from build123d import *

# Parameters (mm, degrees)
SKETCH1_W           = 87
SKETCH1_H           = 90
BOSS_EXTRUDE1_DEPTH = 3
SKETCH2_R           = 3
CUT_EXTRUDE1_DEPTH  = 63.659795723
SKETCH3_R           = 3
CUT_EXTRUDE2_DEPTH  = 63.659795723


with BuildPart() as part:
    # Sketch1 → Boss-Extrude1 (new body)
    with BuildSketch(Plane(origin=(0, 0, 0), x_dir=(1, 0, 0), z_dir=(0, 1, 0))):
        Rectangle(SKETCH1_W, SKETCH1_H)
    extrude(amount=BOSS_EXTRUDE1_DEPTH)

    # Sketch2 → Cut-Extrude1 (cut, through all)
    with BuildSketch(Plane(origin=(0, 3, 0), x_dir=(1, 0, 0), z_dir=(0, 1, 0))):
        with Locations(Location((-18.5, 0, 0), (0, 0, 270))):
            Circle(SKETCH2_R)
    extrude(amount=-CUT_EXTRUDE1_DEPTH, mode=Mode.SUBTRACT)

    # Sketch3 → Cut-Extrude2 (cut, through all)
    with BuildSketch(Plane.XZ):
        with Locations(Location((0, 35, 0), (0, 0, 270))):
            Circle(SKETCH3_R)
        with Locations(Location((-20, -30, 0), (0, 0, 270))):
            Circle(SKETCH3_R)
        with Locations(Location((20, -30, 0), (0, 0, 270))):
            Circle(SKETCH3_R)
    extrude(amount=-CUT_EXTRUDE2_DEPTH, mode=Mode.SUBTRACT)


solid = part.part
Source: CAD feature listing. Evaluate the final solid. Frame: model axes, mm. Give positions to 0.01 mm unless a question says otherwise; leave off trailing zeros. Order: outer loops, then holes, each group sorted by start corner. A loop starts at its lowest first (then second) coordinate and runs counter-clockwise, first axis right, second up. Notation, with made-up numbers: (2.5, 55) -> (33.5, 55) arc R16 cw to (33.5, 71) -> close; hole circle Ø6 at (27.5, -34.75). An arc over 180 degrees is marked (long way). Use a Markdown table: item, result.
1) Section query A-A, the plane x = 0. Return the cut outline in (y, z).
Answer list:
| item | result |
|---|---|
| outline | (0, -45) -> (3, -45) -> (3, 32) -> (0, 32) -> close; (0, 38) -> (3, 38) -> (3, 45) -> (0, 45) -> close |
2) Section query B-B, the plane z = -30. Return the cut outline in (x, y), then the cut area to 3 significant figures.
Answer list:
| item | result |
|---|---|
| outline | (-43.5, 0) -> (-23, 0) -> (-23, 3) -> (-43.5, 3) -> close; (-17, 0) -> (17, 0) -> (17, 3) -> (-17, 3) -> close; (23, 0) -> (43.5, 0) -> (43.5, 3) -> (23, 3) -> close |
| area | 225 mm² |
3) Contact query for a flat-ended pin moving along its axis: P1, Ø5, axis at x = 20, z = -30, coming from the +Y side. Output: stop coordinate, or through.
Answer list:
| item | result |
|---|---|
| P1 | through |
4) Section query C-C, the plane z = 0. Return the cut outline in (x, y).
Answer list:
| item | result |
|---|---|
| outline | (-43.5, 0) -> (-21.5, 0) -> (-21.5, 3) -> (-43.5, 3) -> close; (-15.5, 0) -> (43.5, 0) -> (43.5, 3) -> (-15.5, 3) -> close |
5) Mould query, pull axis Z, two halves, no side actions, for faces 1 (the flat face through (-1, 1, -45)), 2 (the flat face through (-1, 3, -1)), 3 (the cylindrical face through (20, 1, -27)). Classes: +Z half, -Z half, draft (parallel to the pull), parting line (faces both ways), or undercut.
Answer list:
| item | result |
|---|---|
| face 1 | -Z half |
| face 2 | draft |
| face 3 | undercut |
6) Ray query, line 1 along X through (y, z) = (1.45, -30); line 2 along X through (y, z) = (2.2, 35); line 3 along X through (y, z) = (0.7, -2.5). Return the intervals inside material, ascending. Write a range as [from, to].
Answer list:
| item | result |
|---|---|
| line 1 | [-43.5, -23], [-17, 17], [23, 43.5] |
| line 2 | [-43.5, -3], [3, 43.5] |
| line 3 | [-43.5, -20.16], [-16.84, 43.5] |
7) Section query D-D, the plane x = -18.5. Return the cut outline in (y, z).
Answer list:
| item | result |
|---|---|
| outline | (0, -45) -> (3, -45) -> (3, -32.6) -> (0, -32.6) -> close; (0, -27.4) -> (3, -27.4) -> (3, -3) -> (0, -3) -> close; (0, 3) -> (3, 3) -> (3, 45) -> (0, 45) -> close |
